```python
from build123d import *

# Parameters (mm, degrees)
BOSS_EXTRUDE1_DEPTH     = 1.5
CUT_EXTRUDE1_DEPTH      = 52.061237744
CUT_EXTRUDE1_DEPTH_BACK = 52.061237744
SKETCH2_W               = 24
SKETCH2_H               = 24
FILLET1_R               = 5
M2X0_4_TAPPED_HOLE1_D   = 1.6
F_1_5MM_DOWEL_HOLE1_D   = 1.5
FILLET2_R               = 1


with BuildPart() as part:
    # Sketch1 → Boss-Extrude1 (new, symmetric)
    with BuildSketch(Plane(origin=(0, 0, 0), x_dir=(1, 0, 0), z_dir=(0, 1, 0))):
        Polygon((0, 0), (34.748434417, 0), (42, 14.5), (34.748434417, 29), (0, 29), align=None)
    extrude(amount=BOSS_EXTRUDE1_DEPTH, both=True)

    # Sketch2 → Cut-Extrude1 (cut, two sides: drawn at the far end of the back side and taken through both)
    with BuildSketch(Plane(origin=(0, 0, 0), x_dir=(1, 0, 0), z_dir=(0, 1, 0)).offset(-CUT_EXTRUDE1_DEPTH_BACK)):
        with Locations((15, 14.5)):
            Rectangle(SKETCH2_W, SKETCH2_H)
    extrude(amount=CUT_EXTRUDE1_DEPTH + CUT_EXTRUDE1_DEPTH_BACK, mode=Mode.SUBTRACT)

    # Fillet1
    fillet1_edges = [part.edges().sort_by_distance(p)[0] for p in [
        (3, 0, -2.5),
        (3, 0, -26.5),
        (27, 0, -26.5),
        (27, 0, -2.5),
    ]]
    fillet(fillet1_edges, radius=FILLET1_R)

    # M2x0.4 Tapped Hole1 (through all)
    with Locations(Plane(origin=(1.5, 1.5, -27), x_dir=(0, 0, 1), z_dir=(0, 1, 0))):
        with Locations((0, 0), (0, 27), (9.25, 36.248434417), (15.75, 36.248434417), (23, 27), (23, 0)):
            Hole(M2X0_4_TAPPED_HOLE1_D / 2)

    # Ø1.5mm Dowel Hole1 (through all)
    with Locations(Plane(origin=(32.5, 1.5, -16), x_dir=(0, 0, 1), z_dir=(0, 1, 0))):
        with Locations((0, 0), (10, 0)):
            Hole(F_1_5MM_DOWEL_HOLE1_D / 2)

    # Fillet2
    fillet2_edges = [part.edges().sort_by_distance(p)[0] for p in [
        (0, 0, -29),
        (34.748434417, 0, -29),
        (42, 0, -14.5),
        (34.748434417, 0, 0),
        (0, 0, 0),
    ]]
    fillet(fillet2_edges, radius=FILLET2_R)


solid = part.part
```
Verification items for the finished model (mm, model axes). A direction names the side the tool comes from. Give positions to 0.01 mm unless a question says otherwise; leave off trailing zeros. Loops run counter-clockwise (first coordinate to the right, second up) from the corner with the lowest first, then second, coordinate; pieces in that order, holes last. Notation, with made-up numbers: M -18,-17 L 17,-17 A31 ccw 17,13 Z; hole C -20,0.5 d4. An arc over 180 degrees is marked long. Return JSON: item names as keys, results as strings.
1) Tool access check on faces 4 (the flat face through (15, 0, -2.5)), 5 (the flat face through (30, 1.5, -15)). Record the directions out of +Z, -Z, +X, -X, +Y, -Y that give a thin tool (end or side, any length) a straight path to the whole face; none if there is none.
Findings:
{"face 4": "+Y, -Y", "face 5": "+Z, -Z, +X, -X, +Y"}
2) Section check C-C, the plane z = -8.75. Enter the section's corners in (x, y).
Findings:
{"outline": "M 0,-1.5 L 3,-1.5 L 3,1.5 L 0,1.5 Z; M 27,-1.5 L 39.12,-1.5 L 39.12,1.5 L 27,1.5 Z"}
3) Section check B-B, the plane x = 8.5. Enter the section's corners in (y, z), and give its area (3 significant figures).
Findings:
{"outline": "M -1.5,-29 L 1.5,-29 L 1.5,-26.5 L -1.5,-26.5 Z; M -1.5,-2.5 L 1.5,-2.5 L 1.5,0 L -1.5,0 Z", "area": "15.0 mm2"}
4) Gauge pin test, flat end, axial feed: P1, Ø0.9, axis at y = -0.5, z = -15.5, coming from the +X side. Record the tip position at first contact, or that the pin passes through.
Findings:
{"P1": "stops at x = 41.72"}
5) Section check D-D, the plane y = -0.55. Count the separate pieces of the cut face and the enclosed holes in it, and give its area (3 significant figures).
Findings:
{"separate pieces": "1", "enclosed holes": "9", "area": "542 mm2"}
6) Section check A-A, the plane x = 28.5. Enter the section's corners in (y, z).
Findings:
{"outline": "M -1.5,-29 L 1.5,-29 L 1.5,-27.8 L -1.5,-27.8 Z; M -1.5,-26.2 L 1.5,-26.2 L 1.5,-4.8 L -1.5,-4.8 Z; M -1.5,-3.2 L 1.5,-3.2 L 1.5,0 L -1.5,0 Z"}
7) Mould release check, pull along X, two halves, no side actions. Record for faces 1 (the cylindrical face through (0.301, -0.021, -0.285)), 2 (the cylindrical face through (41.88, 0.02, -14.49)), 3 (the cylindrical face through (32.53, -0.02, -15.25)): released by +X, released by -X, zero draft, split by the parting line, or undercut.
Findings:
{"face 1": "released by -X", "face 2": "released by +X", "face 3": "undercut"}
8) Material ranges on L1, parallel to Z at x = 32.5, y = -0.6; L2, parallel to X at y = 0.4, z = -6; L3, parallel to X at y = 0.45, z = -3.5, recorded low to high. Write a range as [from, to].
Findings:
{"L1": "z = [-29, -16.75], [-15.25, -6.75], [-5.25, 0]", "L2": "x = [0, 3.23], [26.77, 31.75], [33.25, 37.75]", "L3": "x = [0, 0.88], [2.12, 5], [25, 27.88], [29.12, 36.5]"}
